from build123d import *

# Parameters (mm, degrees)
CROQUIS1_R              = 1.5
SALIENTE_EXTRUIR1_DEPTH = 4
CROQUIS2_W              = 6.88
CROQUIS2_H              = 20.2
SALIENTE_EXTRUIR2_DEPTH = 5.5
CROQUIS3_R              = 5
CROQUIS3_R_2            = 1.5
SALIENTE_EXTRUIR3_DEPTH = 1.65
CROQUIS4_R              = 1.5
SALIENTE_EXTRUIR4_DEPTH = 1
CROQUIS5_R              = 1.25
CORTAR_EXTRUIR1_DEPTH   = 8


with BuildPart() as part:
    # Croquis1 → Saliente-Extruir1 (new body)
    with BuildSketch(Plane.XY):
        with BuildLine():
            Line((59.9, -8.54), (59.9, 15.2))
            ThreePointArc((59.9, 15.2), (58.435533906, 18.735533906), (54.9, 20.2))
            Line((54.9, 20.2), (40.5, 20.2))
            Line((40.5, 20.2), (40.5, -8.46))
            ThreePointArc((40.5, -8.46), (39.035533906, -11.995533906), (35.5, -13.46))
            Line((35.5, -13.46), (29.128553431, -13.46))
            ThreePointArc((29.128553431, -13.46), (25.5, -11.9), (21.871446569, -13.46))
            Line((21.871446569, -13.46), (0.188553431, -13.46))
            ThreePointArc((0.188553431, -13.46), (0.095533906, -13.364466094), (0, -13.271446569))
            Line((0, -13.271446569), (0, 20.2))
            Line((0, 20.2), (-6.88, 20.2))
            Line((-6.88, 20.2), (-6.88, -13.271446569))
            ThreePointArc((-6.88, -13.271446569), (-6.975533906, -20.435533906), (0.188553431, -20.34))
            Line((0.188553431, -20.34), (21.871446569, -20.34))
            ThreePointArc((21.871446569, -20.34), (25.5, -21.9), (29.128553431, -20.34))
            Line((29.128553431, -20.34), (42.38, -20.34))
            ThreePointArc((42.38, -20.34), (45.915533906, -18.875533906), (47.38, -15.34))
            Line((47.38, -15.34), (47.38, -13.54))
            Line((47.38, -13.54), (54.9, -13.54))
            ThreePointArc((54.9, -13.54), (58.435533906, -12.075533906), (59.9, -8.54))
        make_face()
        with Locations((54.9, 1.74)):
            Circle(CROQUIS1_R, mode=Mode.SUBTRACT)
        with Locations((54.9, -8.54)):
            Circle(CROQUIS1_R, mode=Mode.SUBTRACT)
        with Locations((25.5, -16.9)):
            Circle(CROQUIS1_R, mode=Mode.SUBTRACT)
        with Locations((-3.44, -16.9)):
            Circle(CROQUIS1_R, mode=Mode.SUBTRACT)
        with Locations((54.9, 15.2)):
            Circle(CROQUIS1_R, mode=Mode.SUBTRACT)
    extrude(amount=SALIENTE_EXTRUIR1_DEPTH)

    # Croquis2 → Saliente-Extruir2 (add)
    with BuildSketch(Plane(origin=(0, 0, 0), x_dir=(-1, 0, 0), z_dir=(0, 0, -1))):
        with Locations((-43.94, 10.1)):
            Rectangle(CROQUIS2_W, CROQUIS2_H)
        with Locations((3.44, 10.1)):
            Rectangle(CROQUIS2_W, CROQUIS2_H)
    extrude(amount=SALIENTE_EXTRUIR2_DEPTH)

    # Croquis3 → Saliente-Extruir3 (add)
    with BuildSketch(Plane.XY.offset(4)):
        with Locations(Location((25.5, -16.9, 0), (0, 0, 136.528000689))):
            Circle(CROQUIS3_R)
        with Locations(Location((25.5, -16.9, 0), (0, 0, 249.548360479))):
            Circle(CROQUIS3_R_2, mode=Mode.SUBTRACT)
    extrude(amount=SALIENTE_EXTRUIR3_DEPTH)

    # Croquis4 → Saliente-Extruir4 (add)
    with BuildSketch(Plane(origin=(0, 0, 0), x_dir=(-1, 0, 0), z_dir=(0, 0, -1))):
        with Locations((-25.5, -16.9)):
            Circle(CROQUIS4_R)
        with Locations((-54.9, 1.74)):
            Circle(CROQUIS4_R)
        with Locations((-54.9, -8.54)):
            Circle(CROQUIS4_R)
    extrude(amount=-SALIENTE_EXTRUIR4_DEPTH)

    # Croquis5 → Cortar-Extruir1 (cut)
    with BuildSketch(Plane(origin=(0, 0, -5.5), x_dir=(-1, 0, 0), z_dir=(0, 0, -1))):
        with Locations((-45.5, 5.4)):
            Circle(CROQUIS5_R)
        with Locations((-45.5, 14.8)):
            Circle(CROQUIS5_R)
        with Locations((5, 14.8)):
            Circle(CROQUIS5_R)
        with Locations((5, 5.4)):
            Circle(CROQUIS5_R)
    extrude(amount=-CORTAR_EXTRUIR1_DEPTH, mode=Mode.SUBTRACT)

    # Chaflán1: read off the stored shape, not the designer's step
    # Chaflán1 outline → Chaflán1 (revolve, cut)
    with BuildSketch(Plane(origin=(25.5, -16.9, 0), x_dir=(1, 0, 0), z_dir=(0, -1, 0))):
        Polygon((5, 5.65), (2.401923789, 5.65), (5, 4.15), align=None)
    revolve(axis=Axis((25.5, -16.9, 0), (0, 0, 1)), mode=Mode.SUBTRACT)


solid = part.part
Geometry: final body of the model. Coordinates: model frame, mm. A direction names the side the tool comes from. Coordinates: 2 decimals unless noted, no trailing zeros. Order: outer loops, then holes, each group sorted by start corner. A loop starts at its lowest first (then second) coordinate and runs counter-clockwise, first axis right, second up.
(1) Draft query along X for faces 1 (the face through (55, -9, 1)), 2 (the face through (46, 20.2, 0)). Return one class per face: pulls with the +X half, pulls with the -X half, needs draft (parallel to the pull), parting line crosses it, or undercut.
(2) Material intervals for probe 1 along Y at (x, z) = (45.5, -0.25); probe 2 along X at (y, z) = (11, 3.25); probe 3 along Y at (x, z) = (54.9, 2), sorted ascending.
(3) First-contact query: pin 1 (3.5 mm diameter, centred on x = 54, y = -8, fed in from +Z); pin 2 (4.5 mm diameter, centred on x = 32, z = 1.5, fed in from +Y); pin 3 (5 mm diameter, centred on y = -1, z = -2.5, fed in from -X). Flat tips, straight axial feed; report the tip coordinate or a pass-through.
(4) Section query A-A (z = -2.5). Return the cut outline in (x, y), plus the area to 3 significant figures.
(5) Section query B-B (y = 1.74). Return the cut outline in (x, z).
(6) Section query C-C (x = 10). Return the cut outline in (y, z).
(7) Access query for faces 3 (the face through (34, -15, 0)), 4 (the face through (40.5, 9, -1)), 5 (the face through (46.75, 5.45, -1.56)), 6 (the face through (26, -17, 1)). Directions: +Z, -Z, +X, -X, +Y, -Y. A direction counts if a zero-diameter tool reaches every point of the face in a straight line with its end or side. Return the directions, or none.
(8) Section query D-D (x = 49). Return the cut outline in (y, z).
Solution:
1. face 1: undercut
1. face 2: needs draft
2. probe 1: y = 0 to 4.15, 6.65 to 13.55, 16.05 to 20.2
2. probe 2: x = -6.88 to 0, 40.5 to 59.9
2. probe 3: y = -13.54 to -10.04, -7.04 to 0.24, 3.24 to 13.7, 16.7 to 20.2
3. pin 1: stops at z = 4
3. pin 2: stops at y = -13.46
3. pin 3: stops at x = -6.88
4. outline: (-6.88, 0) - (0, 0) - (0, 20.2) - (-6.88, 20.2) - close; (40.5, 0) - (47.38, 0) - (47.38, 20.2) - (40.5, 20.2) - close; hole circle Ø2.5 at (-5, 5.4); hole circle Ø2.5 at (-5, 14.8); hole circle Ø2.5 at (45.5, 5.4); hole circle Ø2.5 at (45.5, 14.8)
4. area: 258 mm2
5. outline: (-6.88, -5.5) - (0, -5.5) - (0, 4) - (-6.88, 4) - close; (40.5, -5.5) - (47.38, -5.5) - (47.38, 0) - (59.9, 0) - (59.9, 4) - (56.4, 4) - (56.4, 1) - (53.4, 1) - (53.4, 4) - (40.5, 4) - close
6. outline: (-20.34, 0) - (-13.46, 0) - (-13.46, 4) - (-20.34, 4) - close
7. face 3: -Z, +X, -Y
7. face 4: +Z, -Z, +Y
7. face 5: -Z
7. face 6: +Z
8. outline: (-13.54, 0) - (20.2, 0) - (20.2, 4) - (-13.54, 4) - close
